Geometry check sheet. Reference: the model listing, model coordinates, mm. A direction names the side the tool comes from. Round coordinates to 2 decimals unless told otherwise and drop trailing zeros. Loops run counter-clockwise (first coordinate to the right, second up) from the corner with the lowest first, then second, coordinate; pieces in that order, holes last.
```python
from build123d import *

# Parameters (mm, degrees)
CROQUIS1_W              = 10
CROQUIS1_H              = 4
SALIENTE_EXTRUIR1_DEPTH = 15
CROQUIS2_R              = 1.5
CORTAR_EXTRUIR1_DEPTH   = 15


with BuildPart() as part:
    # Croquis1 → Saliente-Extruir1 (new body)
    with BuildSketch(Plane(origin=(0, 0, 0), x_dir=(1, 0, 0), z_dir=(0, 1, 0))):
        Polygon((-8.75, 3.25), (-8.75, -7.25), (8.75, -7.25), (8.75, 7.25), (6.75, 7.25), (6.75, -5.592857143), (-6.75, -5.592857143), (-6.75, 7.25), (-8.75, 7.25), align=None)
        with Locations((-13.75, 5.25)):
            Rectangle(CROQUIS1_W, CROQUIS1_H)
    extrude(amount=SALIENTE_EXTRUIR1_DEPTH)

    # Croquis2 → Cortar-Extruir1 (cut)
    with BuildSketch(Plane.XY.offset(-3.25)):
        with Locations((-13.75, 7.5)):
            Circle(CROQUIS2_R)
    extrude(amount=-CORTAR_EXTRUIR1_DEPTH, mode=Mode.SUBTRACT)


solid = part.part
```
1) Access from +Z, -Z, +X, -X, +Y, -Y to the whole of each face (thin tool, end or side, straight path). Record for faces 1 (the face through (8, 7, -7.25)), 2 (the face through (6.75, 7, -1)).
Report:
face 1: -Z, +X, -X, +Y, -Y
face 2: -Z, +Y, -Y
2) Sectioned sample at D-D, the plane y = 3. Record the cut outline in (x, z).
Report:
outline: (-18.75, -7.25) - (-6.75, -7.25) - (-6.75, 5.59) - (6.75, 5.59) - (6.75, -7.25) - (8.75, -7.25) - (8.75, 7.25) - (-8.75, 7.25) - (-8.75, -3.25) - (-18.75, -3.25) - close
3) Sectioned sample at B-B, the plane x = -13.75. Record the cut outline in (y, z).
Report:
outline: (0, -7.25) - (6, -7.25) - (6, -3.25) - (0, -3.25) - close; (9, -7.25) - (15, -7.25) - (15, -3.25) - (9, -3.25) - close
4) Sectioned sample at A-A, the plane y = 7.5. Record the cut outline in (x, z), then the cut area to 3 significant figures.
Report:
outline: (-18.75, -7.25) - (-15.25, -7.25) - (-15.25, -3.25) - (-18.75, -3.25) - close; (-12.25, -7.25) - (-6.75, -7.25) - (-6.75, 5.59) - (6.75, 5.59) - (6.75, -7.25) - (8.75, -7.25) - (8.75, 7.25) - (-8.75, 7.25) - (-8.75, -3.25) - (-12.25, -3.25) - close
area: 108 mm2
5) Sectioned sample at C-C, the plane z = -0.75. Record the cut outline in (x, y).
Report:
outline: (-8.75, 0) - (-6.75, 0) - (-6.75, 15) - (-8.75, 15) - close; (6.75, 0) - (8.75, 0) - (8.75, 15) - (6.75, 15) - close
6) Mould release check, pull along X, two halves, no side actions. Record for faces 3 (the face through (-8.75, 7, 2)), 4 (the face through (0, 7, 5.593)), 5 (the face through (-13.8, 5.7, -3.25)): +X half, -X half, draft (parallel to the pull), parting line (faces both ways), or undercut.
Report:
face 3: -X half
face 4: undercut
face 5: draft
7) Scan lines: line 1 along X through (y, z) = (13.5, -5.5); line 2 along Y through (x, z) = (-13.75, -5.55); line 3 along X through (y, z) = (6.75, -4.25). Record each from-to range of solid material in increasing order.
Report:
line 1: x = -18.75 to -6.75, 6.75 to 8.75
line 2: y = 0 to 6, 9 to 15
line 3: x = -18.75 to -15.05, -12.45 to -6.75, 6.75 to 8.75
8) Gauge pin test, flat ends, axial feed: pin 1 (6 mm diameter, centred on x = -1.5, z = -3, fed in from +Y); pin 2 (8.5 mm diameter, centred on y = 7.5, z = 2.5, fed in from -X); pin 3 (3 mm diameter, centred on x = 5.5, z = -1, fed in from +Y); pin 4 (5 mm diameter, centred on x = -13, y = 10.5, fed in from +Z). Record the tip position at first contact, or that the pin passes through.
Report:
pin 1: passes through
pin 2: stops at x = -8.75
pin 3: stops at y = 15
pin 4: stops at z = -3.25
